Design review of the part built by this model. Coordinates are the model's own, in mm. Face numbers are marked on the shaded views. A direction names the side the tool comes from. Coordinates: 2 decimals unless noted, no trailing zeros. Loops run counter-clockwise (first coordinate to the right, second up) from the corner with the lowest first, then second, coordinate; pieces in that order, holes last.
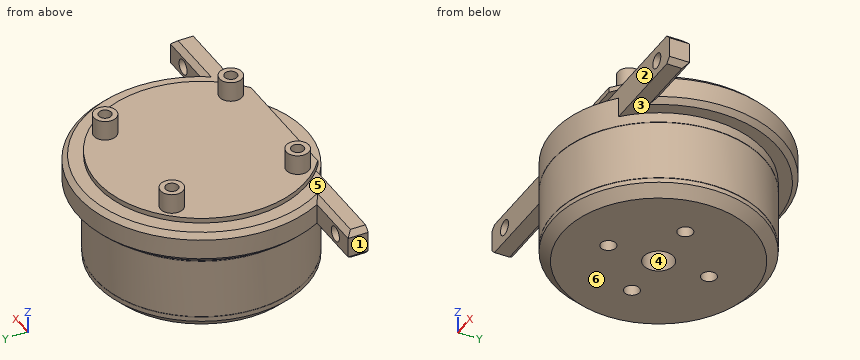
from build123d import *

# Parameters (mm, degrees)
SKETCH1_R               = 21
BOSS_EXTRUDE1_DEPTH     = 3
CHAMFER1_SIZE           = 2
FILLET1_R               = 0.1
SKETCH2_R               = 21
BOSS_EXTRUDE2_DEPTH     = 12
FILLET2_R               = 0.1
SKETCH3_R               = 21
BOSS_EXTRUDE3_DEPTH     = 6
SKETCH4_R               = 3
SKETCH4_R_2             = 1.5
CUT_EXTRUDE1_DEPTH      = 6
BOSS_EXTRUDE4_DEPTH     = 6
CHAMFER2_SIZE           = 1
CUT_EXTRUDE2_DEPTH      = 55.134670037
CUT_EXTRUDE2_DEPTH_BACK = 55.134670037
SKETCH6_R               = 1.5
BOSS_EXTRUDE5_DEPTH     = 1
SKETCH8_R               = 2.25
BOSS_EXTRUDE6_DEPTH     = 4
SKETCH9_R               = 1.25
CUT_EXTRUDE3_DEPTH      = 4


with BuildPart() as part:
    # Sketch1 → Boss-Extrude1 (new body)
    with BuildSketch(Plane.XY):
        Circle(SKETCH1_R)
    extrude(amount=BOSS_EXTRUDE1_DEPTH)

    # Chamfer1
    chamfer1_edges = [part.edges().sort_by_distance(p)[0] for p in [
        (-21, 0, 0),
    ]]
    chamfer(chamfer1_edges, length=CHAMFER1_SIZE)

    # Fillet1
    fillet1_edges = [part.edges().sort_by_distance(p)[0] for p in [
        (-21, 0, 3),
    ]]
    fillet(fillet1_edges, radius=FILLET1_R)

    # Sketch2 → Boss-Extrude2 (add)
    with BuildSketch(Plane.XY.offset(3)):
        Circle(SKETCH2_R)
    extrude(amount=BOSS_EXTRUDE2_DEPTH)

    # Fillet2
    fillet2_edges = [part.edges().sort_by_distance(p)[0] for p in [
        (-21, 0, 15),
    ]]
    fillet(fillet2_edges, radius=FILLET2_R)

    # Sketch3 → Boss-Extrude3 (add)
    with BuildSketch(Plane.XY.offset(15)):
        Circle(SKETCH3_R)
    extrude(amount=BOSS_EXTRUDE3_DEPTH)

    # Sketch4 → Cut-Extrude1 (cut)
    with BuildSketch(Plane(origin=(0, 0, 0), x_dir=(-1, 0, 0), z_dir=(0, 0, -1))):
        Circle(SKETCH4_R)
        with Locations((-10, 0)):
            Circle(SKETCH4_R_2)
        with Locations((0, 10)):
            Circle(SKETCH4_R_2)
        with Locations((10, 0)):
            Circle(SKETCH4_R_2)
        with Locations((0, -10)):
            Circle(SKETCH4_R_2)
    extrude(amount=-CUT_EXTRUDE1_DEPTH, mode=Mode.SUBTRACT)

    # Sketch5 → Boss-Extrude4 (add)
    with BuildSketch(Plane.XY.offset(17)):
        with BuildLine():
            Line((21.633307653, -11.5), (33.25, -11.5))
            Line((33.25, -11.5), (33.25, -15.5))
            Line((33.25, -15.5), (-33.25, -15.5))
            Line((-33.25, -15.5), (-33.25, -11.5))
            Line((-33.25, -11.5), (-21.633307653, -11.5))
            ThreePointArc((-21.633307653, -11.5), (0, 24.5), (21.633307653, -11.5))
        make_face()
    extrude(amount=BOSS_EXTRUDE4_DEPTH)

    # Chamfer2
    chamfer2_edges = [part.edges().sort_by_distance(p)[0] for p in [
        (0, 24.5, 17),
        (-27.441653826, -11.5, 17),
        (-33.25, -13.5, 17),
        (33.25, -13.5, 17),
        (27.441653826, -11.5, 17),
        (0, 24.5, 23),
        (-27.441653826, -11.5, 23),
        (-33.25, -13.5, 23),
        (33.25, -13.5, 23),
        (27.441653826, -11.5, 23),
    ]]
    chamfer(chamfer2_edges, length=CHAMFER2_SIZE)

    # Sketch6 → Cut-Extrude2 (cut, two sides: drawn at the far end of the back side and taken through both)
    with BuildSketch(Plane(origin=(0, -11.5, 0), x_dir=(1, 0, 0), z_dir=(0, 1, 0)).offset(-CUT_EXTRUDE2_DEPTH_BACK)):
        with Locations(Location((-28.5, -20, 0), (0, 0, 180))):
            Circle(SKETCH6_R)
        with Locations(Location((28.5, -20, 0), (0, 0, 180))):
            Circle(SKETCH6_R)
    extrude(amount=CUT_EXTRUDE2_DEPTH + CUT_EXTRUDE2_DEPTH_BACK, mode=Mode.SUBTRACT)

    # Sketch7 → Boss-Extrude5 (add)
    with BuildSketch(Plane.XY.offset(23)):
        with BuildLine():
            Line((12.499599994, -16.5), (-12.499599994, -16.5))
            ThreePointArc((-12.499599994, -16.5), (0, 20.7), (12.499599994, -16.5))
        make_face()
    extrude(amount=BOSS_EXTRUDE5_DEPTH)

    # Sketch8 → Boss-Extrude6 (add)
    with BuildSketch(Plane.XY.offset(24)):
        with Locations((-12.5, 12.5)):
            Circle(SKETCH8_R)
        with Locations((12.5, 12.5)):
            Circle(SKETCH8_R)
        with Locations((12.5, -12.5)):
            Circle(SKETCH8_R)
        with Locations((-12.5, -12.5)):
            Circle(SKETCH8_R)
    extrude(amount=BOSS_EXTRUDE6_DEPTH)

    # Sketch9 → Cut-Extrude3 (cut)
    with BuildSketch(Plane.XY.offset(28)):
        with Locations((12.5, 12.5)):
            Circle(SKETCH9_R)
        with Locations((12.5, -12.5)):
            Circle(SKETCH9_R)
        with Locations((-12.5, 12.5)):
            Circle(SKETCH9_R)
        with Locations((-12.5, -12.5)):
            Circle(SKETCH9_R)
    extrude(amount=-CUT_EXTRUDE3_DEPTH, mode=Mode.SUBTRACT)


solid = part.part
Q1. For line 1 (Y direction, x = -12.5, z = 25.05); line 2 (X direction, y = -12.7, z = 20); line 3 (Y direction, x = 0, z = 4.6), list the stretches that pass through material, from the lowest coordinate up.
Q2. Take a section at B-B, the plane x = -28.5. Write out the cut boundary in (y, z), then the cut area to 3 significant figures.
Q3. The part is to be moulded in two halves that separate along Z. For the marked faces 1, 2 and 3, say which applies: pulls with the +Z half, pulls with the -Z half, needs draft (parallel to the pull), parting line crosses it, or undercut.
Q4. Clearance check with flat-ended pins moving along their axes: pin 1 Ø1 at (x, y) = (3.5, 13.5) entering from +Z; pin 2 Ø1.2 at (x, z) = (25.5, 20) entering from +Y; pin 3 Ø5 at (x, z) = (-16.5, 5) entering from -Y. State where each tip first meets the part, or that it passes through.
Q5. Machinability: for the marked faces 4, 5 and 6, which of the approach directions +Z, -Z, +X, -X, +Y, -Y give a long, thin tool a straight path to every point of the face, cutting with its end or side? Answer none if there is none.
Q6. Take a section at A-A, the plane z = 20. Write out the cut boundary in (x, y).
Entries:
1. line 1: y = -14.75 to -13.75, -11.25 to -10.25, 10.25 to 11.25, 13.75 to 14.75
1. line 2: x = -33.25 to -30, -27 to 27, 30 to 33.25
1. line 3: y = -21 to -11.5, -8.5 to -3, 3 to 8.5, 11.5 to 21
2. outline: (-15.5, 17) - (-12.5, 17) - (-11.5, 18) - (-11.5, 18.5) - (-15.5, 18.5) - close; (-15.5, 21.5) - (-11.5, 21.5) - (-11.5, 22) - (-12.5, 23) - (-15.5, 23) - close
2. area: 11.0 mm2
3. face 1: needs draft
3. face 2: undercut
3. face 3: pulls with the -Z half
4. pin 1: stops at z = 24
4. pin 2: stops at y = -11.5
4. pin 3: stops at y = -15.65
5. face 4: -Z
5. face 5: +Z
5. face 6: -Z, +X, -X, +Y, -Y
6. outline: (-33.25, -15.5) - (-30, -15.5) - (-30, -11.5) - (-33.25, -11.5) - close; (-27, -15.5) - (-14.17, -15.5) arc R21 ccw to (14.17, -15.5) - (27, -15.5) - (27, -11.5) - (21.63, -11.5) arc R24.5 ccw (long way) to (-21.63, -11.5) - (-27, -11.5) - close; (30, -15.5) - (33.25, -15.5) - (33.25, -11.5) - (30, -11.5) - close
